Geometry: final body of the model. Coordinates: model frame, mm. A direction names the side the tool comes from. Give positions to 0.01 mm unless a question says otherwise; leave off trailing zeros. Write each loop counter-clockwise with the first axis right and the second up, starting at its lowest first coordinate (ties: lowest second). Pieces come first, ordered by that corner, then holes.
from build123d import *

# Parameters (mm, degrees)
SKETCH_1_R          = 3.5
EXTRUDE_1_DEPTH     = 3.9
SKETCH_2_R          = 2
EXTRUDE_2_DEPTH     = 35
CUT_EXTRUDE_1_DEPTH = 2.4


with BuildPart() as part:
    # 草图1 → 凸台-拉伸1 (new body)
    with BuildSketch(Plane(origin=(0, 0, 0), x_dir=(1, 0, 0), z_dir=(0, 1, 0))):
        Circle(SKETCH_1_R)
    extrude(amount=EXTRUDE_1_DEPTH)

    # 草图2 → 凸台-拉伸2 (add)
    with BuildSketch(Plane(origin=(0, 3.9, 0), x_dir=(1, 0, 0), z_dir=(0, 1, 0))):
        Circle(SKETCH_2_R)
    extrude(amount=EXTRUDE_2_DEPTH)

    # 草图3 → 切除-拉伸1 (cut)
    with BuildSketch(Plane.XZ):
        Polygon((1.725, 0), (0.8625, 1.493893822), (-0.8625, 1.493893822), (-1.725, 0), (-0.8625, -1.493893822), (0.8625, -1.493893822), align=None)
    extrude(amount=-CUT_EXTRUDE_1_DEPTH, mode=Mode.SUBTRACT)


solid = part.part
Q1. Pin query (flat end, axial travel): P1, Ø2, axis at x = -2.5, y = 31.5, coming from the +Z side; P2, Ø0.9, axis at x = 0.5, z = 0, coming from the -Y side; P3, Ø2, axis at y = 8.5, z = -0.5, coming from the -X side. Return the tip coordinate at first contact, or that it passes through.
Filled sheet:
P1: stops at z = 1.32
P2: stops at y = 2.4
P3: stops at x = -2
Q2. Section B-B on y = 30. Output: boundary loops of the cut face in (x, z), plus the area to 3 significant figures.
Filled sheet:
outline: circle Ø4 at (0, 0)
area: 12.6 mm2
Q3. Pull-direction query (X, two-part tool) for faces 4 (the flat face through (-1.288, 1.183, 0.757)), 5 (the flat face through (0, 38.9, 0)), 6 (the cylindrical face through (0, 21, 2)); classes: released by +X, released by -X, zero draft, split by the parting line, or undercut.
Filled sheet:
face 4: undercut
face 5: zero draft
face 6: split by the parting line
Q4. Section C-C on x = -3. Output: boundary loops of the cut face in (y, z).
Filled sheet:
outline: (0, -1.8) - (3.9, -1.8) - (3.9, 1.8) - (0, 1.8) - close
Q5. Ray query, line 1 along X through (y, z) = (25, -1); line 2 along Y through (x, z) = (-2.25, -0.5); line 3 along Y through (x, z) = (-1.25, -0.5). Return the intervals inside material, ascending.
Filled sheet:
line 1: x = -1.73 to 1.73
line 2: y = 0 to 3.9
line 3: y = 2.4 to 38.9
Q6. Access query for faces 1 (the flat face through (2, 3.9, 2)), 2 (the flat face through (0, 2.4, 0)), 3 (the flat face through (0, 0, 2)). Directions: +Z, -Z, +X, -X, +Y, -Y. A direction counts if a zero-diameter tool reaches every point of the face in a straight line with its end or side. Return the directions, or none.
Filled sheet:
face 1: +Y
face 2: -Y
face 3: +Z, -Z, +X, -X, -Y
Q7. Section A-A on x = 0. Output: boundary loops of the cut face in (y, z), plus the area to 3 significant figures.
Filled sheet:
outline: (0, -3.5) - (3.9, -3.5) - (3.9, -2) - (38.9, -2) - (38.9, 2) - (3.9, 2) - (3.9, 3.5) - (0, 3.5) - (0, 1.49) - (2.4, 1.49) - (2.4, -1.49) - (0, -1.49) - close
area: 160 mm2
